from build123d import *

# Parameters (mm, degrees)
F1_DEPTH = 50
F3_DEPTH = 25
F4_R     = 5


# Not quite as in the source:
# - a feature names something its author has since deleted; it is built from what else it names


with BuildPart() as f1:
    # F0 (on Front) → F1 (new body)
    with BuildSketch(Plane.XZ):
        Polygon((0, 0), (0, -2), (20, -2), (20, -90), (22, -90), (22, 10), (20, 10), (20, 0), align=None)
    extrude(amount=F1_DEPTH)

    # F2 (on face) → F3 (cut)
    with BuildSketch(Plane.XY):
        with BuildLine():
            ThreePointArc((12, -7), (10, -5), (8, -7))
            Line((8, -7), (8, -13))
            ThreePointArc((8, -13), (10, -15), (12, -13))
            Line((12, -13), (12, -7))
        make_face()
        with BuildLine():
            ThreePointArc((8, -43), (10, -45), (12, -43))
            Line((12, -43), (12, -37))
            ThreePointArc((12, -37), (10, -35), (8, -37))
            Line((8, -37), (8, -43))
        make_face()
    extrude(amount=-F3_DEPTH, mode=Mode.SUBTRACT)

    # F4
    f4_edges = [f1.edges().sort_by_distance(p)[0] for p in [
        (21, -50, 10),
        (21, 0, 10),
        (21, -50, -90),
        (21, 0, -90),
        (0, -50, -1),
        (0, 0, -1),
    ]]
    fillet(f4_edges, radius=F4_R)


solid = f1.part
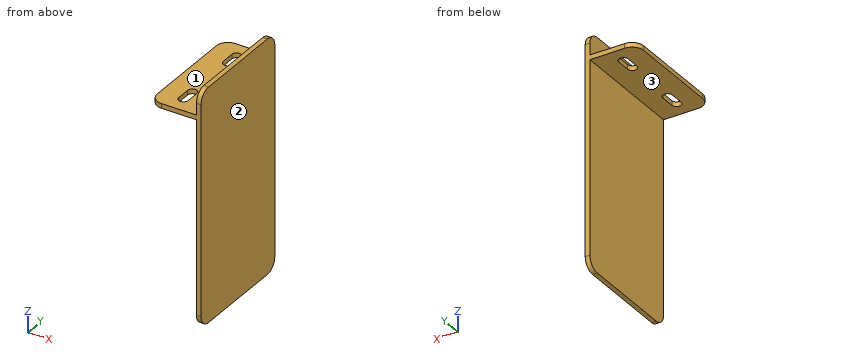
Can you work these out from the model? Positions are in its coordinate system, mm. Face numbers are marked on the shaded views. A direction names the side the tool comes from. Give positions to 0.01 mm unless a question says otherwise; leave off trailing zeros. Loops run counter-clockwise (first coordinate to the right, second up) from the corner with the lowest first, then second, coordinate; pieces in that order, holes last. Notation, with made-up numbers: M 43.5,5.25 L 58.5,5.25 A17 ccw 58.5,13.25 Z; hole C 60.25,56 d5. An arc over 180 degrees is marked long. One line per item, written item: value. Start each with the question number.
1) I'm going to push flat-ended pins straight in: pin 1 (6 mm diameter, centred on x = 6, y = -16.5, fed in from -Z); pin 2 (12 mm diameter, centred on y = -8.5, z = -25, fed in from -X); pin 3 (10 mm diameter, centred on x = 6.5, y = -15, fed in from +Z). Where does each tip first touch, or does it pass through?
2) If we section it at D-D, the plane z = -58.5: Write out the boundary of the cut face in (x, y), and give its area (3 significant figures).
3) If we section it at C-C, the plane y = -33.5: Write out the boundary of the cut face in (x, z).
4) If we section it at A-A, the plane x = 10: Write out the boundary of the cut face in (y, z).
5) On a 3-axis mill with a long thin cutter (end or side, diameter ignored), from which of +Z, -Z, +X, -X, +Y, -Y can I reach the whole of each face in a straight line? I mean the marked faces 1, 2 and 3. Say none if no direction works.
6) If I drill on line 1 (X direction, y = -31, z = -61); line 2 (Z direction, x = 9, y = -20), over which ranges is the centre line in solid material (lowest first)? Write a range as [from, to].
7) If we section it at B-B, the plane y = -12: Write out the boundary of the cut face in (x, z), and give its area (3 significant figures).
Completed:
1. pin 1: stops at z = -2
1. pin 2: stops at x = 20
1. pin 3: stops at z = 0
2. outline: M 20,-50 L 22,-50 L 22,0 L 20,0 Z
2. area: 100 mm^2
3. outline: M 0,-2 L 20,-2 L 20,-90 L 22,-90 L 22,10 L 20,10 L 20,0 L 0,0 Z
4. outline: M -50,-2 L -45,-2 L -45,0 L -50,0 Z; M -35,-2 L -15,-2 L -15,0 L -35,0 Z; M -5,-2 L 0,-2 L 0,0 L -5,0 Z
5. face 1: +Z, -X, +Y, -Y
5. face 2: +Z, -Z, +X, +Y, -Y
5. face 3: -Z, -X, +Y, -Y
6. line 1: x = [20, 22]
6. line 2: z = [-2, 0]
7. outline: M 0,-2 L 8,-2 L 8,0 L 0,0 Z; M 12,-2 L 20,-2 L 20,-90 L 22,-90 L 22,10 L 20,10 L 20,0 L 12,0 Z
7. area: 232 mm^2
